Read the model definition and answer for the solid it produces. Units are mm, in the model's axes. A direction names the side the tool comes from. Give positions to 0.01 mm unless a question says otherwise; leave off trailing zeros. Order: outer loops, then holes, each group sorted by start corner. A loop starts at its lowest first (then second) coordinate and runs counter-clockwise, first axis right, second up. Notation, with made-up numbers: (50, -24) - (102, -24) arc R18 ccw to (102, -9) - close; hole circle Ø11 at (-31, 34.5). An arc over 180 degrees is marked (long way). Use a Markdown table: item, result. Add a question column.
1. A cutting plane is placed at B-B on y = 0. Determine the outline of the cut face in (x, z).
2. A cutting plane is placed at A-A on z = 0. Determine the outline of the cut face in (x, y).
3. Which of the six approach directions +Z, -Z, +X, -X, +Y, -Y give full straight-line access (tool end or side, diameter ignored) to faces 1 (the cylindrical face through (24.971, -1.802, 5.723)), 2 (the flat face through (3.6, 0, 0))?
4. Consider L1, parallel to Y at x = 2.5, z = -0.25; L2, parallel to Z at x = 19.5, y = -0.25; L3, parallel to Y at x = 4, z = -3.25. Determine where each line is inside the solid, lowest interval first.
5. Flat-ended cylindrical pins translate along their axes: P1, Ø4, axis at x = 5.5, z = 2.5, coming from the -Y side; P2, Ø5, axis at x = 21, y = 4, coming from the -Z side; P3, Ø2, axis at x = 40, y = -1.5, coming from the +Z side. Find the tip coordinate at first contact, or state that the pin passes through.
6. A cutting plane is placed at C-C on x = 44.5. Determine the outline of the cut face in (y, z).
7. For a pull along Y with two mould halves and no side action, classify faces 3 (the conical face through (0.097, 5.202, -0.102)), 4 (the flat face through (2, 1, 0)), 5 (the flat face through (0, -3, 0)) as released by +Y, released by -Y, zero draft, split by the parting line, or undercut.
```python
from build123d import *

# Parameters (mm, degrees)
SKETCH2_W  = 12
SKETCH2_H  = 2
SLOT_DEPTH = 3.6


with BuildPart() as part:
    # BodySke → BaseBody (revolve)
    with BuildSketch(Plane.XY, mode=Mode.PRIVATE) as basebody_sk:
        with BuildLine():
            Line((0.556565659, 6), (48.711457479, 6))
            ThreePointArc((48.711457479, 6), (49.674233358, 3.068401124), (50, 0))
            Line((50, 0), (0, 0))
            Line((0, 0), (0, 5.036))
            Line((0, 5.036), (0.556565659, 6))
        make_face()
    revolve(basebody_sk.sketch.rotate(Axis((-12.7, 0, 0), (1, 0, 0)), 90), axis=Axis((-12.7, 0, 0), (1, 0, 0)))

    # Sketch2 → Slot (cut)
    with BuildSketch(Plane(origin=(0, 0, 0), x_dir=(0, 0, -1), z_dir=(1, 0, 0))):
        Rectangle(SKETCH2_W, SKETCH2_H)
    extrude(amount=SLOT_DEPTH, mode=Mode.SUBTRACT)


solid = part.part
```
Output values:
| question | item | result |
|---|---|---|
| 1 | outline | (3.6, -6) - (48.71, -6) arc R14.61 ccw to (48.71, 6) - (3.6, 6) - close |
| 2 | outline | (0, -5.04) - (0.56, -6) - (48.71, -6) arc R14.61 ccw to (48.71, 6) - (0.56, 6) - (0, 5.04) - (0, 1) - (3.6, 1) - (3.6, -1) - (0, -1) - close |
| 3 | face 1 | +X, -X |
| 3 | face 2 | +Z, -Z, -X |
| 4 | L1 | -5.99 to -1, 1 to 5.99 |
| 4 | L2 | -5.99 to 5.99 |
| 4 | L3 | -5.04 to 5.04 |
| 5 | P1 | y = -5.98 |
| 5 | P2 | z = -5.81 |
| 5 | P3 | z = 5.98 |
| 6 | outline | circle Ø12 at (0, 0) |
| 7 | face 3 | released by +Y |
| 7 | face 4 | undercut |
| 7 | face 5 | zero draft |
